The figure shows three views and two pictorial views of one solid part (mm, origin at its lowest corner). Answer the questions. A direction names the side the tool comes from. Round coordinates to 2 decimals unless told otherwise and drop trailing zeros. Loops run counter-clockwise (first coordinate to the right, second up) from the corner with the lowest first, then second, coordinate; pieces in that order, holes last. Notation, with made-up numbers: (-30, 26.5) -> (25, 26.5) arc R21 ccw to (25, 58.5) -> close; hole circle Ø10 at (-35.75, 17). An arc over 180 degrees is marked (long way). Use a Markdown table: item, result. Add a question column.
Q1. Consider line 1 (X direction, y = 48, z = 26); line 2 (Y direction, x = 68.35, z = 18); line 3 (Y direction, x = 16.5, z = 29). Determine where each line is inside the solid, lowest interval first.
Q2. Section D-D on z = 8 is taken. Give the vertices of the cut face in (x, y), then the cut area to 3 significant figures.
Q3. Given pin 1 Ø12 at (x, y) = (55.5, 8.5) entering from -Z; pin 2 Ø11 at (x, z) = (6.5, 21) entering from -Y; pin 3 Ø4 at (y, z) = (1.5, 16) entering from +X, each flat-ended and moving along its own axis, determine where each tip first touches the part or whether it passes through.
Q4. Which of the six approach directions +Z, -Z, +X, -X, +Y, -Y give full straight-line access (tool end or side, diameter ignored) to the marked faces 1, 2, 3, 4 and 5?
Q5. Section A-A on z = 18 is taken. Give the vertices of the cut face in (x, y).
Q6. Section B-B on y = 35 is taken. Give the vertices of the cut face in (x, z), then the cut area to 3 significant figures.
Q7. For a pull along X with two mould halves and no side action, classify the marked faces 6, 7, 8 and 9 as released by +X, released by -X, zero draft, split by the parting line, or undercut.
Q8. Section C-C on y = 15.5 is taken. Give the vertices of the cut face in (x, z), then the cut area to 3 significant figures.
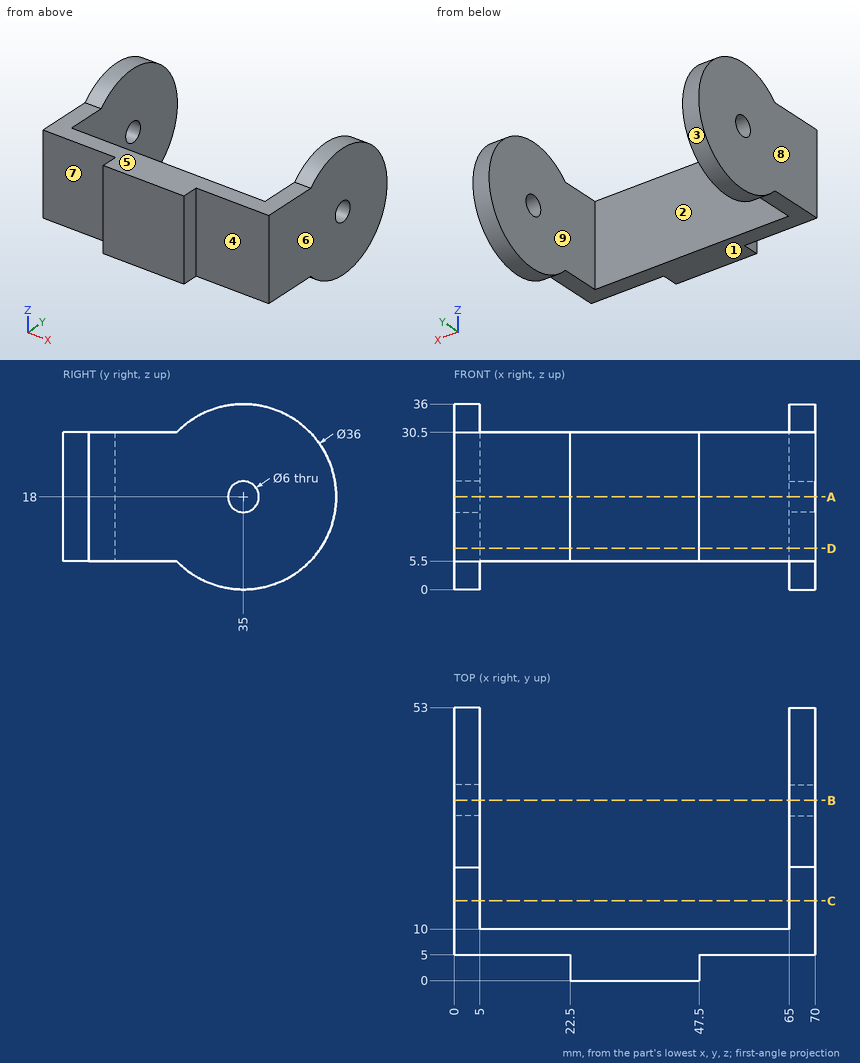
Checked values:
| question | item | result |
|---|---|---|
| 1 | line 1 | x = 0 to 5, 65 to 70 |
| 1 | line 2 | y = 5 to 32, 38 to 53 |
| 1 | line 3 | y = 5 to 10 |
| 2 | outline | (0, 5) -> (22.5, 5) -> (22.5, 0) -> (47.5, 0) -> (47.5, 5) -> (70, 5) -> (70, 49.97) -> (65, 49.97) -> (65, 10) -> (5, 10) -> (5, 49.97) -> (0, 49.97) -> close |
| 2 | area | 875 mm2 |
| 3 | pin 1 | stops at z = 5.5 |
| 3 | pin 2 | stops at y = 5 |
| 3 | pin 3 | stops at x = 47.5 |
| 4 | face 1 | -Z, +X, -X, -Y |
| 4 | face 2 | +Z, -Z, +Y |
| 4 | face 3 | +X, -X |
| 4 | face 4 | +Z, -Z, +X, -Y |
| 4 | face 5 | +Z, +X, -X, -Y |
| 5 | outline | (0, 5) -> (22.5, 5) -> (22.5, 0) -> (47.5, 0) -> (47.5, 5) -> (70, 5) -> (70, 32) -> (65, 32) -> (65, 10) -> (5, 10) -> (5, 32) -> (0, 32) -> close; (0, 38) -> (5, 38) -> (5, 53) -> (0, 53) -> close; (65, 38) -> (70, 38) -> (70, 53) -> (65, 53) -> close |
| 6 | outline | (0, 0) -> (5, 0) -> (5, 15) -> (0, 15) -> close; (0, 21) -> (5, 21) -> (5, 36) -> (0, 36) -> close; (65, 0) -> (70, 0) -> (70, 15) -> (65, 15) -> close; (65, 21) -> (70, 21) -> (70, 36) -> (65, 36) -> close |
| 6 | area | 300 mm2 |
| 7 | face 6 | released by +X |
| 7 | face 7 | zero draft |
| 7 | face 8 | released by -X |
| 7 | face 9 | undercut |
| 8 | outline | (0, 5.5) -> (5, 5.5) -> (5, 30.5) -> (0, 30.5) -> close; (65, 5.5) -> (70, 5.5) -> (70, 30.5) -> (65, 30.5) -> close |
| 8 | area | 250 mm2 |
